Job drawing, mm, ordinate dimensions from the low corner. One solid piece. A direction names the side the tool comes from. Give positions to 0.01 mm unless a question says otherwise; leave off trailing zeros. Loops run counter-clockwise (first coordinate to the right, second up) from the corner with the lowest first, then second, coordinate; pieces in that order, holes last. Notation, with made-up numbers: (67, 30.25) -> (78, 30.25) arc R33 cw to (78, 69.25) -> close; hole circle Ø1 at (88, 64.25). An arc over 180 degrees is marked (long way). Answer as a JSON object with one key per item and string values. Group by question number.
Q1. Tool access for the marked faces 1 and 2: list every direction of +Z, -Z, +X, -X, +Y, -Y with a clear straight run to the whole face (end or side of a thin tool).
Q2. Band-saw the part on B-B, the plane x = 32.5. Write the cut outline in (y, z), plus the area to 3 significant figures.
Q3. Band-saw the part on A-A, the plane y = 13.5. Write the cut outline in (x, z).
Q4. Band-saw the part on C-C, the plane z = 16.25. Count the separate pieces of the cut face and the enclosed holes in it, plus the area to 3 significant figures.
Q5. Band-saw the part on D-D, the plane x = 40. Write the cut outline in (y, z).
Q6. Wall check: probe 1 along X at (y, z) = (1.55, 15); probe 2 along Y at (x, z) = (8.5, 21); probe 3 along X at (y, z) = (3.5, 15). Give the ranges that are in metal, low to high. Write a range as from..to.
Q7. Drop flat-ended pins along their axis: pin 1 (14 mm diameter, centred on x = 13.5, z = 22, fed in from +Y); pin 2 (3 mm diameter, centred on x = 5, z = 15, fed in from +Y); pin 3 (6 mm diameter, centred on y = 8.5, z = 24.5, fed in from -X); pin 4 (3.5 mm diameter, centred on x = 44.5, z = 9, fed in from +Y). Give the stop position or say it passes through.
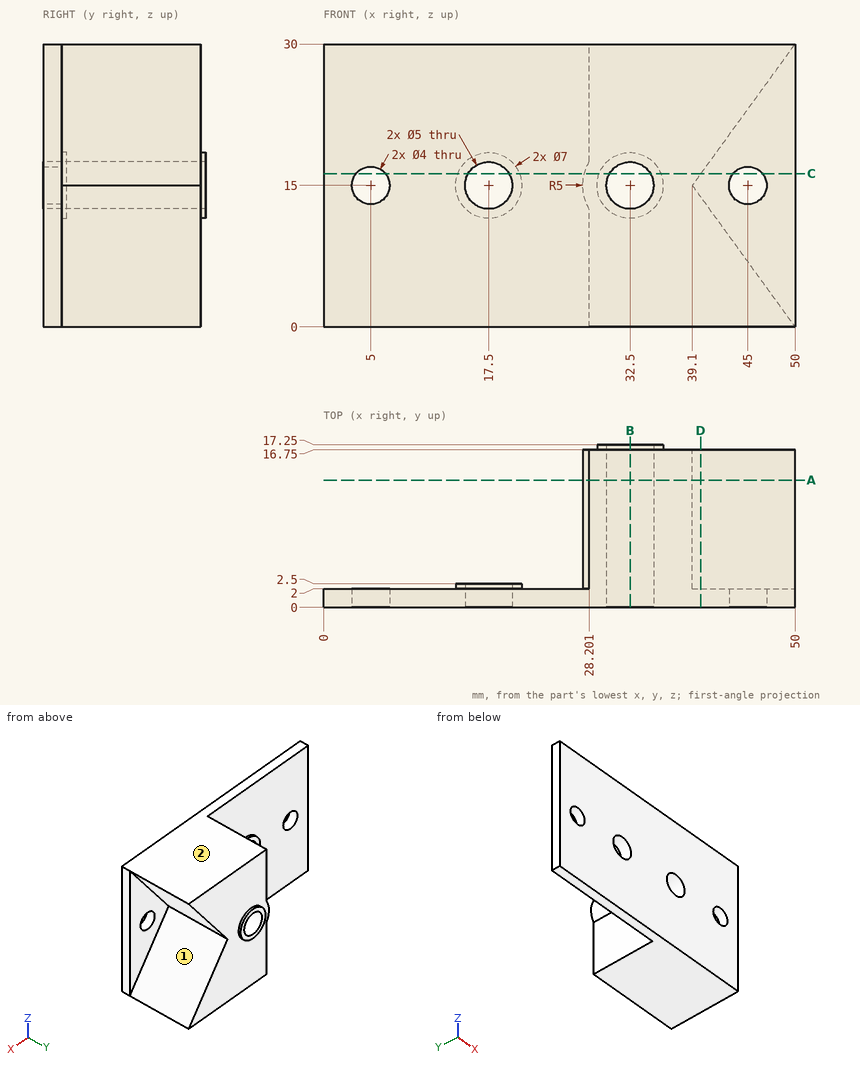
Worked answers:
{
 "1": {"face 1": "+X, +Y", "face 2": "+Z, +X, -X, +Y, -Y"},
 "2": {"outline": "(0, 0) -> (16.75, 0) -> (16.75, 11.5) -> (17.25, 11.5) -> (17.25, 12.5) -> (0, 12.5) -> close; (0, 17.5) -> (17.25, 17.5) -> (17.25, 18.5) -> (16.75, 18.5) -> (16.75, 30) -> (0, 30) -> close", "area": "420 mm2"},
 "3": {"outline": "(28.2, 0) -> (50, 0) -> (39.1, 15) -> (50, 30) -> (28.2, 30) -> (28.2, 17.55) arc R5 ccw to (28.2, 12.45) -> close; hole circle Ø5 at (32.5, 15)"},
 "4": {"separate pieces": "5", "enclosed holes": "0", "area": "191 mm2"},
 "5": {"outline": "(0, 0) -> (16.75, 0) -> (16.75, 13.76) -> (2, 13.76) -> (2, 16.24) -> (16.75, 16.24) -> (16.75, 30) -> (0, 30) -> close"},
 "6": {"probe 1": "0..3, 7..15, 20..30, 35..43, 47..50", "probe 2": "0..2", "probe 3": "27.5..30, 35..39.1"},
 "7": {"pin 1": "y = 2.5", "pin 2": "through", "pin 3": "x = 28.2", "pin 4": "y = 16.75"}
}
